```python
from build123d import *

# Parameters (mm, degrees)
SKETCH_1_W           = 90
SKETCH_1_H           = 25
EXTRUDE_1_DEPTH      = 15
CUT_EXTRUDE_1_DEPTH  = 15
SKETCH_3_R           = 2.5
CUT_EXTRUDE_2_DEPTH  = 15
SKETCH_4_W           = 1.8
SKETCH_4_H           = 7
CUT_EXTRUDE_3_DEPTH  = 5
SKETCH_5_R           = 1.65
CUT_EXTRUDE_4_DEPTH  = 5
SKETCH_6_W           = 20
SKETCH_6_H           = 2.5
CUT_EXTRUDE_5_DEPTH  = 5
CUT_EXTRUDE_7_DEPTH  = 7.5
CUT_EXTRUDE_8_DEPTH  = 7.5
SKETCH_9_R           = 2
SKETCH_9_W           = 8
SKETCH_9_H           = 4
EXTRUDE_2_DEPTH      = 1
FILLET_1_R           = 2
CUT_EXTRUDE_10_REACH = 51.369
SKETCH_15_W          = 17.204453114
SKETCH_15_H          = 35.420932882


with BuildPart() as part:
    # 草图1 → 凸台-拉伸1 (new body)
    with BuildSketch(Plane.XY):
        Rectangle(SKETCH_1_W, SKETCH_1_H)
    extrude(amount=EXTRUDE_1_DEPTH)

    # 草图2 → 切除-拉伸1 (cut)
    with BuildSketch(Plane.XY.offset(15)):
        with BuildLine():
            Line((-32.5, 12.5), (-61.464378833, 12.5))
            Line((-61.464378833, 12.5), (-61.464378833, -12.5))
            Line((-61.464378833, -12.5), (-32.5, -12.5))
            ThreePointArc((-32.5, -12.5), (-45, 0), (-32.5, 12.5))
        make_face()
        with BuildLine():
            Line((32.5, 12.5), (60.882590951, 12.5))
            Line((60.882590951, 12.5), (60.882590951, -12.5))
            Line((60.882590951, -12.5), (32.5, -12.5))
            ThreePointArc((32.5, -12.5), (45, 0), (32.5, 12.5))
        make_face()
    extrude(amount=-CUT_EXTRUDE_1_DEPTH, mode=Mode.SUBTRACT)

    # 草图3 → 切除-拉伸2 (cut)
    with BuildSketch(Plane(origin=(0, 12.5, 0), x_dir=(1, 0, 0), z_dir=(0, 1, 0))):
        with Locations(Location((0, -7.5, 0), (0, 0, 180))):
            Circle(SKETCH_3_R)
    extrude(amount=-CUT_EXTRUDE_2_DEPTH, mode=Mode.SUBTRACT)

    # 草图4 → 切除-拉伸3 (cut)
    with BuildSketch(Plane(origin=(0, 12.5, 0), x_dir=(1, 0, 0), z_dir=(0, 1, 0))):
        with Locations((-8.384632086, -7.5)):
            Rectangle(SKETCH_4_W, SKETCH_4_H)
        with Locations((-5.384632086, -7.5)):
            Rectangle(SKETCH_4_W, SKETCH_4_H)
        with Locations((-11.384632086, -7.5)):
            Rectangle(SKETCH_4_W, SKETCH_4_H)
        with Locations((-14.384632086, -7.5)):
            Rectangle(SKETCH_4_W, SKETCH_4_H)
        with Locations((-17.384632086, -7.5)):
            Rectangle(SKETCH_4_W, SKETCH_4_H)
        with Locations((-20.384632086, -7.5)):
            Rectangle(SKETCH_4_W, SKETCH_4_H)
        with Locations((-23.384632086, -7.5)):
            Rectangle(SKETCH_4_W, SKETCH_4_H)
        with Locations((-26.384632086, -7.5)):
            Rectangle(SKETCH_4_W, SKETCH_4_H)
        with Locations((-29.384632086, -7.5)):
            Rectangle(SKETCH_4_W, SKETCH_4_H)
        with Locations((-32.384632086, -7.5)):
            Rectangle(SKETCH_4_W, SKETCH_4_H)
    cut_extrude_3 = extrude(amount=-CUT_EXTRUDE_3_DEPTH, mode=Mode.SUBTRACT)

    # 镜向1: 切除-拉伸3 across plane
    add(cut_extrude_3.mirror(Plane(origin=(0, 0, 0), x_dir=(0, 0, 1), z_dir=(1, 0, 0))), mode=Mode.SUBTRACT)

    # 草图5 → 切除-拉伸4 (cut)
    with BuildSketch(Plane(origin=(0, 0, 0), x_dir=(-1, 0, 0), z_dir=(0, 0, -1))):
        with Locations((-22.5, 0)):
            Circle(SKETCH_5_R)
        with Locations((22.5, 0)):
            Circle(SKETCH_5_R)
    extrude(amount=-CUT_EXTRUDE_4_DEPTH, mode=Mode.SUBTRACT)

    # 草图6 → 切除-拉伸5 (cut)
    with BuildSketch(Plane.XZ.offset(12.5)):
        with Locations((0, 2.5)):
            Rectangle(SKETCH_6_W, SKETCH_6_H)
    extrude(amount=-CUT_EXTRUDE_5_DEPTH, mode=Mode.SUBTRACT)

    # 草图7 → 切除-拉伸7 (cut)
    with BuildSketch(Plane(origin=(0, 0, 0), x_dir=(-1, 0, 0), z_dir=(0, 0, -1))):
        with BuildLine():
            Line((-32.5, 9), (-32.5, -9))
            ThreePointArc((-32.5, -9), (-41.5, 0), (-32.5, 9))
        make_face()
    extrude(amount=-CUT_EXTRUDE_7_DEPTH, mode=Mode.SUBTRACT)

    # 草图8 → 切除-拉伸8 (cut)
    with BuildSketch(Plane(origin=(32.5, 0, 0), x_dir=(0, 0, -1), z_dir=(1, 0, 0))):
        with BuildLine():
            Line((-1.91780044, -4), (-1.91780044, 4))
            ThreePointArc((-1.91780044, 4), (-2.91780044, 5), (-3.91780044, 4))
            Line((-3.91780044, 4), (-3.91780044, -4))
            ThreePointArc((-3.91780044, -4), (-2.91780044, -5), (-1.91780044, -4))
        make_face()
    extrude(amount=-CUT_EXTRUDE_8_DEPTH, mode=Mode.SUBTRACT)

    # 草图9 → 凸台-拉伸2 (add)
    with BuildSketch(Plane.XY.offset(15)):
        with Locations((28, 0)):
            Circle(SKETCH_9_R)
        with Locations((-26.5, 0)):
            Circle(SKETCH_9_R)
        with Locations((-40.5, 0)):
            Circle(SKETCH_9_R)
        with Locations((1, 0)):
            Rectangle(SKETCH_9_W, SKETCH_9_H)
    extrude(amount=EXTRUDE_2_DEPTH)

    # 圆角1
    # the kernel refuses this fillet: 2 mm, written as the material it takes off along each edge
    with BuildSketch(Plane(origin=(32.5, -12.5, 0), x_dir=(0, 0, 1), z_dir=(-1, 0, 0))) as fillet_1_piece_1:
        with BuildLine():
            CenterArc((FILLET_1_R, FILLET_1_R), FILLET_1_R, 180, 90)
            Line((0, FILLET_1_R), (0, 0))
            Line((0, 0), (FILLET_1_R, 0))
        make_face()
    extrude(amount=65, mode=Mode.SUBTRACT)
    with BuildSketch(Plane(origin=(-32.5, 0, 0), x_dir=(0, -1, 0), z_dir=(1, 0, 0))) as fillet_1_piece_2:
        with BuildLine():
            CenterArc((12.5 - FILLET_1_R, -FILLET_1_R), FILLET_1_R, 0, 90)
            Line((12.5, -FILLET_1_R), (12.5, 0))
            Line((12.5, 0), (12.5 - FILLET_1_R, 0))
        make_face()
    revolve(axis=Axis((-32.5, 0, 0), (0, 0, -1)), revolution_arc=180, mode=Mode.SUBTRACT)
    with BuildSketch(Plane(origin=(-32.5, 12.5, 0), x_dir=(0, -1, 0), z_dir=(1, 0, 0))) as fillet_1_piece_3:
        with BuildLine():
            CenterArc((FILLET_1_R, -FILLET_1_R), FILLET_1_R, 90, 90)
            Line((0, -FILLET_1_R), (0, 0))
            Line((0, 0), (FILLET_1_R, 0))
        make_face()
    extrude(amount=65, mode=Mode.SUBTRACT)
    with BuildSketch(Plane(origin=(32.5, 0, 0), x_dir=(0, 1, 0), z_dir=(-1, 0, 0))) as fillet_1_piece_4:
        with BuildLine():
            CenterArc((12.5 - FILLET_1_R, -FILLET_1_R), FILLET_1_R, 0, 90)
            Line((12.5, -FILLET_1_R), (12.5, 0))
            Line((12.5, 0), (12.5 - FILLET_1_R, 0))
        make_face()
    revolve(axis=Axis((32.5, 0, 0), (0, 0, -1)), revolution_arc=180, mode=Mode.SUBTRACT)

    # 切除-拉伸10: up to this face of the body (flat: up to its plane)
    cut_extrude_10_end = Plane(part.part.faces().sort_by_distance((36.351487084, -0.076382797, 7.5))[0])
    # 草图15 → 切除-拉伸10 (cut, up to the picked face)
    with BuildSketch(Plane(origin=(0, 0, 0), x_dir=(-1, 0, 0), z_dir=(0, 0, -1)), mode=Mode.PRIVATE) as cut_extrude_10_sk1:
        with Locations((-40.69229177, 2.139850544)):
            Rectangle(SKETCH_15_W, SKETCH_15_H)
    cut_extrude_10_tool1 = split(extrude(cut_extrude_10_sk1.sketch, amount=-CUT_EXTRUDE_10_REACH, mode=Mode.PRIVATE), bisect_by=cut_extrude_10_end, keep=Keep.BOTH, mode=Mode.PRIVATE)
    add(cut_extrude_10_tool1.solids().sort_by(Axis((40.692292, 2.139851, 0), (0, 0, 1)))[0], mode=Mode.SUBTRACT)


solid = part.part
```
Build history of the part. All positions in model axes, mm. A direction names the side the tool comes from. Round coordinates to 2 decimals unless told otherwise and drop trailing zeros. Loops run counter-clockwise (first coordinate to the right, second up) from the corner with the lowest first, then second, coordinate; pieces in that order, holes last.
Item 1: Drill centre lines: line 1 along Z through (x, y) = (0, 7); line 2 along Z through (x, y) = (21, -3); line 3 along Z through (x, y) = (-2, 7.25). Where is each one in solid material? Low to high.
Item 2: Two-plate mould, pull along Y, no slides. Class faces 6 (the face through (11, 7.5, 7)), 7 (the face through (-20.85, 0.07, 2.46)), 8 (the face through (24.285, 10, 8)): released by +Y, released by -Y, zero draft, split by the parting line, or undercut.
Item 3: Which spindle directions (+Z, -Z, +X, -X, +Y, -Y) get a long thin tool onto all of the face, cutting with end or side? Do faces 1 (the face through (29, 0, 1.918)), 2 (the face through (-10, -10, 2)), 3 (the face through (45, 0, 11)), 4 (the face through (-42.498, 0.088, 15.493)), 5 (the face through (-31.485, 10, 8)). Say none if no direction does.
Item 4: Pin check, flat tips, straight feed: P1, Ø6.5, axis at x = 37.5, y = -1, coming from the -Z side; P2, Ø2, axis at x = -1, z = 2.5, coming from the -Y side; P3, Ø8, axis at y = 5.5, z = 4, coming from the +X side. Stop position of each tip, or through.
Item 5: Saw through at A-A (x = 0). List the corners of the cut face in (y, z), then the cut area to 3 significant figures.
Worked answers:
1. line 1: z = 0 to 5, 10 to 15
1. line 2: z = 0 to 15
1. line 3: z = 0 to 6, 9 to 15
2. face 6: released by +Y
2. face 7: undercut
2. face 8: zero draft
3. face 1: +X
3. face 2: -Y
3. face 3: +Z, -Z, +X
3. face 4: +Z
3. face 5: +Y
4. P1: stops at z = 7.5
4. P2: stops at y = -7.5
4. P3: stops at x = 44.48
5. outline: (-12.5, 3.75) - (-7.5, 3.75) - (-7.5, 1.25) - (-12.35, 1.25) arc R2 ccw to (-10.5, 0) - (10.5, 0) arc R2 ccw to (12.5, 2) - (12.5, 5) - (-2.5, 5) - (-2.5, 10) - (12.5, 10) - (12.5, 15) - (2, 15) - (2, 16) - (-2, 16) - (-2, 15) - (-12.5, 15) - close
5. area: 290 mm2
